```python
from build123d import *

# Parameters (mm, degrees)
BOSS_EXTRUDE1_DEPTH      = 30
BOSS_EXTRUDE1_DEPTH_BACK = 30
SKETCH2_W                = 74
SKETCH2_H                = 39
SKETCH2_W_2              = 70
SKETCH2_H_2              = 35
CUT_EXTRUDE1_DEPTH       = 65.171644829
CUT_EXTRUDE1_DEPTH_BACK  = 65.171644829
SKETCH1_R                = 1.25
SKETCH1_R_2              = 2.5
CUT_EXTRUDE2_START       = -37
CUT_EXTRUDE2_DEPTH       = 74
SKETCH4_R                = 1.75
CUT_EXTRUDE3_DEPTH       = 3
SKETCH5_R                = 1.5
SKETCH5_W                = 3.5
SKETCH5_H                = 19.9
CUT_EXTRUDE4_DEPTH       = 61.3158354


# Read off the part's stored shape, not the designer's step: Cut-Extrude2
with BuildPart() as part:
    # Sketch2 → Boss-Extrude1 (new, two sides: drawn at the far end of the back side and taken through both)
    with BuildSketch(Plane(origin=(0, 0, 0), x_dir=(0, 0, -1), z_dir=(1, 0, 0)).offset(-BOSS_EXTRUDE1_DEPTH_BACK)):
        with Locations((0, 23.5)):
            Rectangle(SKETCH2_W, SKETCH2_H)
        with Locations((0, 23.5)):
            Rectangle(SKETCH2_W_2, SKETCH2_H_2, mode=Mode.SUBTRACT)
    extrude(amount=BOSS_EXTRUDE1_DEPTH + BOSS_EXTRUDE1_DEPTH_BACK)

    # Sketch1 → Cut-Extrude1 (cut, two sides: drawn at the far end of the back side and taken through both)
    with BuildSketch(Plane.XY.offset(-CUT_EXTRUDE1_DEPTH_BACK)):
        with Locations((8.5, 20)):
            Circle(SKETCH1_R)
        with Locations((-8.5, 20)):
            Circle(SKETCH1_R)
        with Locations((0, 10)):
            Circle(SKETCH1_R_2)
    extrude(amount=CUT_EXTRUDE1_DEPTH + CUT_EXTRUDE1_DEPTH_BACK, mode=Mode.SUBTRACT)

    # Cut-Extrude2 outline → Cut-Extrude2 (cut)
    with BuildSketch(Plane.XY.offset(CUT_EXTRUDE2_START)):
        Polygon((-6.223385238, 23), (6.291063493, 23), (0.075182746, 29.257087778), align=None)
        Polygon((-13.493003356, 24.235644043), (-4.153418424, 33.513721677), (-10.100273174, 39.5), (-26.5, 39.5), (-26.5, 37.242640687), align=None)
        Polygon((10.385998459, 39.5), (4.331816644, 33.485688948), (13.507019797, 24.249660484), (26.5, 37.242640687), (26.5, 39.5), align=None)
        Polygon((21.757359313, 7.5), (13.5, 15.757359313), (5.242640687, 7.5), align=None)
        Polygon((26.5, 28.757359313), (17.742640687, 20), (26.5, 11.242640687), align=None)
        Polygon((-13.5, 15.757359313), (-21.757359313, 7.5), (-5.242640687, 7.5), align=None)
        with BuildLine():
            Line((2.432627089, 13.175267776), (6.257359313, 17))
            Line((6.257359313, 17), (-6.257359313, 17))
            Line((-6.257359313, 17), (-2.432627089, 13.175267776))
            ThreePointArc((-2.432627089, 13.175267776), (0, 14), (2.432627089, 13.175267776))
        make_face()
        Polygon((-26.5, 11.242640687), (-17.742640687, 20), (-26.5, 28.757359313), align=None)
        Polygon((1.872544824, 39.5), (-1.642886221, 39.5), (0.103215475, 37.742322846), align=None)
    extrude(amount=CUT_EXTRUDE2_DEPTH, mode=Mode.SUBTRACT)

    # Sketch4 → Cut-Extrude3 (cut)
    with BuildSketch(Plane(origin=(0, 43, 0), x_dir=(1, 0, 0), z_dir=(0, 1, 0))):
        with Locations(Location((-20, 27, 0), (0, 0, 270))):
            Circle(SKETCH4_R)
        with Locations(Location((20, 27, 0), (0, 0, 270))):
            Circle(SKETCH4_R)
        with Locations(Location((20, -27, 0), (0, 0, 270))):
            Circle(SKETCH4_R)
        with Locations(Location((-20, -27, 0), (0, 0, 270))):
            Circle(SKETCH4_R)
    extrude(amount=-CUT_EXTRUDE3_DEPTH, mode=Mode.SUBTRACT)

    # Sketch5 → Cut-Extrude4 (cut, through all)
    with BuildSketch(Plane(origin=(0, 6, 0), x_dir=(1, 0, 0), z_dir=(0, 1, 0))):
        with Locations(Location((-26.460092097, -18.5, 0), (0, 0, 270))):
            Circle(SKETCH5_R)
        with Locations(Location((-26.460092097, 18.5, 0), (0, 0, 270))):
            Circle(SKETCH5_R)
        with Locations(Location((10.539907903, 18.5, 0), (0, 0, 270))):
            Circle(SKETCH5_R)
        with Locations(Location((10.539907903, -18.5, 0), (0, 0, 270))):
            Circle(SKETCH5_R)
        with Locations(Location((28, -7.75, 0), (0, 0, 270))):
            Circle(SKETCH5_R)
        with Locations(Location((28, 7.75, 0), (0, 0, 270))):
            Circle(SKETCH5_R)
        with Locations((16.25, 0)):
            Rectangle(SKETCH5_W, SKETCH5_H)
    extrude(amount=-CUT_EXTRUDE4_DEPTH, mode=Mode.SUBTRACT)


solid = part.part
```
CAD build for the part. Positions are in the model's coordinates, mm. A direction names the side the tool comes from. Give positions to 0.01 mm unless a question says otherwise; leave off trailing zeros. Write each loop counter-clockwise with the first axis right and the second up, starting at its lowest first coordinate (ties: lowest second). Pieces come first, ordered by that corner, then holes. Notation, with made-up numbers: (83, 17.25) -> (128, 17.25) arc R29 cw to (128, 56.25) -> close; hole circle Ø10 at (30.25, -37). An arc over 180 degrees is marked (long way). Write each question's results on one line, items separated by ' | '.
1. Cut at D-D, the plane z = -32. Write the cut outline in (x, y), then the cut area to 3 significant figures.
Geometry check:
outline: (-30, 4) -> (30, 4) -> (30, 6) -> (-30, 6) -> close; (-30, 41) -> (30, 41) -> (30, 43) -> (-30, 43) -> close | area: 240 mm²
2. Wall check: probe 1 along X at (y, z) = (42.35, -27); probe 2 along X at (y, z) = (5.3, -7.75); probe 3 along Y at (x, z) = (26, 3). Give the ranges that are in metal, low to high. Write a range as [from, to].
Geometry check:
probe 1: [-30, -21.75], [-18.25, 18.25], [21.75, 30] | probe 2: [-30, 14.5], [18, 26.5], [29.5, 30] | probe 3: [4, 6], [41, 43]
3. Which spindle directions (+Z, -Z, +X, -X, +Y, -Y) get a long thin tool onto all of the face, cutting with end or side? Do faces 1 (the cylindrical face through (10.6, 5, -20)), 2 (the cylindrical face through (21.18, 42.01, 25.71)), 3 (the flat face through (13, 7.5, -36)). Say none if no direction does.
Geometry check:
face 1: -Y | face 2: +Y | face 3: +Z, -Z
4. Drop flat-ended pins along their axis: P1, Ø4, axis at x = 0, y = 10, coming from the +Z side; P2, Ø2.5, axis at x = -26.46, z = 18.5, coming from the -Y side. Give the stop position or say it passes through.
Geometry check:
P1: through | P2: y = 41
5. Cut at C-C, the plane y = 8.5. Give the number of separate pieces and of enclosed holes in the cut face, then the cut area to 3 significant figures.
Geometry check:
separate pieces: 8 | enclosed holes: 0 | area: 108 mm²
6. Cut at A-A, the plane z = 27. Write the cut outline in (x, y).
Geometry check:
outline: (-30, 4) -> (30, 4) -> (30, 6) -> (-30, 6) -> close; (-30, 41) -> (-21.75, 41) -> (-21.75, 43) -> (-30, 43) -> close; (-18.25, 41) -> (18.25, 41) -> (18.25, 43) -> (-18.25, 43) -> close; (21.75, 41) -> (30, 41) -> (30, 43) -> (21.75, 43) -> close
7. Cut at B-B, the plane x = 28. Write the cut outline in (y, z), then the cut area to 3 significant figures.
Geometry check:
outline: (4, -37) -> (43, -37) -> (43, 37) -> (4, 37) -> (4, 9.25) -> (6, 9.25) -> (6, 35) -> (41, 35) -> (41, -35) -> (6, -35) -> (6, -9.25) -> (4, -9.25) -> close; (4, -6.25) -> (6, -6.25) -> (6, 6.25) -> (4, 6.25) -> close | area: 424 mm²
8. Two-plate mould, pull along X, no slides. Class faces 4 (the flat face through (8.86, 28.93, -36.01)), 5 (the cylindrical face through (0, 14, 36)), 6 (the flat face through (0, 6, 0)): pulls with the +X half, pulls with the -X half, needs draft (parallel to the pull), parting line crosses it, or undercut.
Geometry check:
face 4: undercut | face 5: undercut | face 6: needs draft
